```python
from build123d import *

# Parameters (mm, degrees)
SKETCH_3_R               = 2.5
SKETCH_3_R_2             = 1.375
SKETCH_3_R_3             = 0.625
EXTRUDE_1_DEPTH          = 12
CUT_EXTRUDE_START        = -6
SKETCH_4_R               = 1.375
SKETCH_4_R_2             = 0.625
CUT_EXTRUDE_1_DEPTH      = 6
CUT_EXTRUDE_2_DEPTH      = 6
CUT_EXTRUDE_3_DEPTH      = 98.323451249
CUT_EXTRUDE_3_DEPTH_BACK = 98.323451249
SKETCH_9_W               = 7.034569735
SKETCH_9_H               = 2.5


with BuildPart() as part:
    # 草图3 → 凸台-拉伸1 (new body)
    # profile 1 of 4: a face of its own
    with BuildSketch(Plane.XY):
        with BuildLine():
            ThreePointArc((-61.260434814, -42.25), (-62.911250508, -39.426764685), (-66.181254237, -39.480854503))
            Line((-66.181254237, -39.480854503), (-67.215081256, -40.482765899))
            ThreePointArc((-67.215081256, -40.482765899), (-66.804847725, -44.526501605), (-62.766497887, -44.986741313))
            ThreePointArc((-62.766497887, -44.986741313), (-61.661816101, -43.8118882), (-61.260434814, -42.25))
        make_face()
        with Locations((-64.5, -42.25)):
            Circle(SKETCH_3_R, mode=Mode.SUBTRACT)
    # profile 2 of 4: a face of its own
    with BuildSketch(Plane.XY):
        with BuildLine():
            ThreePointArc((-62.766497887, -44.986741313), (-66.804847725, -44.526501605), (-67.215081256, -40.482765899))
            Line((-67.215081256, -40.482765899), (-71.404577544, -44.542926834))
            Line((-71.404577544, -44.542926834), (-68.869512223, -46.563873564))
            ThreePointArc((-68.869512223, -46.563873564), (-68.283195443, -46.88782244), (-67.622796748, -47))
            Line((-67.622796748, -47), (-65.944900832, -47))
            Line((-65.944900832, -47), (-62.766497887, -44.986741313))
        make_face()
    # profile 3 of 4: a face of its own
    with BuildSketch(Plane.XY):
        with Locations((-78.5, -53.325)):
            Circle(SKETCH_3_R_2)
        with Locations((-78.5, -53.325)):
            Circle(SKETCH_3_R_3, mode=Mode.SUBTRACT)
    # profile 4 of 4: a face of its own
    with BuildSketch(Plane.XY):
        with BuildLine():
            Line((-68.869512223, -46.563873564), (-71.404577544, -44.542926834))
            Line((-71.404577544, -44.542926834), (-79.356399518, -52.24926543))
            ThreePointArc((-79.356399518, -52.24926543), (-77.902892111, -52.086417274), (-77.125, -53.325))
            ThreePointArc((-77.125, -53.325), (-77.295362144, -53.987927323), (-77.764232924, -54.486581598))
            Line((-77.764232924, -54.486581598), (-65.944900832, -47))
            Line((-65.944900832, -47), (-67.622796748, -47))
            ThreePointArc((-67.622796748, -47), (-68.283195443, -46.88782244), (-68.869512223, -46.563873564))
        make_face()
    extrude(amount=EXTRUDE_1_DEPTH)

    # 草图4 → 切除-拉伸1 (cut)
    with BuildSketch(Plane.XY.offset(6).offset(CUT_EXTRUDE_START)):
        with Locations((-78.5, -53.325)):
            Circle(SKETCH_4_R)
        with Locations((-78.5, -53.325)):
            Circle(SKETCH_4_R_2, mode=Mode.SUBTRACT)
    extrude(amount=CUT_EXTRUDE_1_DEPTH, mode=Mode.SUBTRACT)

    # 草图5 → 切除-拉伸2 (cut)
    with BuildSketch(Plane(origin=(0, 0, 0), x_dir=(-1, 0, 0), z_dir=(0, 0, -1))):
        with BuildLine():
            Line((79.356399518, -52.24926543), (78.605866383, -51.521902256))
            ThreePointArc((78.605866383, -51.521902256), (78.66209541, -51.603950043), (78.681882496, -51.701428318))
            ThreePointArc((78.681882496, -51.701428318), (78.612326251, -51.874460255), (78.442362088, -51.951208578))
            ThreePointArc((78.442362088, -51.951208578), (78.926279835, -52.017746963), (79.356399518, -52.24926543))
        make_face()
        with BuildLine():
            Line((79.691485429, -51.10916302), (78.328547162, -51.10916302))
            Line((78.328547162, -51.10916302), (78.328547162, -51.253144251))
            Line((78.328547162, -51.253144251), (78.605866383, -51.521902256))
            Line((78.605866383, -51.521902256), (79.356399518, -52.24926543))
            ThreePointArc((79.356399518, -52.24926543), (78.926279835, -52.017746963), (78.442362088, -51.951208578))
            ThreePointArc((78.442362088, -51.951208578), (78.385355708, -51.954787722), (78.328547162, -51.960731359))
            Line((78.328547162, -51.960731359), (78.328547162, -52.568011757))
            Line((78.328547162, -52.568011757), (79.691485429, -52.568011757))
            Line((79.691485429, -52.568011757), (79.691485429, -51.10916302))
        make_face()
        with BuildLine():
            Line((76.773632808, -53.859117327), (76.559713092, -53.723616657))
            Line((76.559713092, -53.723616657), (76.559713092, -54.626372146))
            Line((76.559713092, -54.626372146), (77.832544784, -54.626372146))
            Line((77.832544784, -54.626372146), (77.832544784, -53.006023906))
            Line((77.832544784, -53.006023906), (77.162510093, -53.006023906))
            ThreePointArc((77.162510093, -53.006023906), (77.125199423, -53.301582625), (77.152422696, -53.598240569))
            ThreePointArc((77.152422696, -53.598240569), (77.36758294, -54.104908073), (77.764232924, -54.486581598))
            Line((77.764232924, -54.486581598), (76.773632808, -53.859117327))
        make_face()
        with BuildLine():
            ThreePointArc((77.152422696, -53.598240569), (77.049210108, -53.853814684), (76.773632808, -53.859117327))
            Line((76.773632808, -53.859117327), (77.764232924, -54.486581598))
            ThreePointArc((77.764232924, -54.486581598), (77.36758294, -54.104908073), (77.152422696, -53.598240569))
        make_face()
    extrude(amount=-CUT_EXTRUDE_2_DEPTH, mode=Mode.SUBTRACT)

    # 草图9 → 切除-拉伸3 (cut, two sides: drawn at the far end of the back side and taken through both)
    with BuildSketch(Plane(origin=(-4.269265018, 5.396813566, 0), x_dir=(-0.784272958804573, -0.6204159299114752, 0), z_dir=(0.6204159299114752, -0.784272958804573, 0)).offset(-CUT_EXTRUDE_3_DEPTH_BACK)):
        with Locations((76.928026692, -1.25)):
            Rectangle(SKETCH_9_W, SKETCH_9_H)
        Polygon((74.298785761, -9.5), (73.410741824, -9.5), (73.410741824, -12), (80.445311559, -12), (80.445311559, -9.5), align=None)
    extrude(amount=CUT_EXTRUDE_3_DEPTH + CUT_EXTRUDE_3_DEPTH_BACK, mode=Mode.SUBTRACT)


solid = part.part
```
Verification items for the finished model (mm, model axes). A direction names the side the tool comes from. Coordinates: 2 decimals unless noted, no trailing zeros. Write each loop counter-clockwise with the first axis right and the second up, starting at its lowest first coordinate (ties: lowest second). Pieces come first, ordered by that corner, then holes. Notation, with made-up numbers: M 27,74.25 L 53,74.25 A25 cw 53,91.25 Z; hole C -23,12 d10. An arc over 180 degrees is marked long. One line per item, written item: value.
Item 1: Section check A-A, the plane x = -63.25. Record the boundary of the cut face in (y, z), plus the area to 3 significant figures.
Check sheet entries:
outline: M -45.29,2.5 L -44.42,2.5 L -44.42,9.5 L -45.29,9.5 Z; M -40.08,2.5 L -39.26,2.5 L -39.26,9.5 L -40.08,9.5 Z
area: 11.9 mm^2
Item 2: Access from +Z, -Z, +X, -X, +Y, -Y to the whole of each face (thin tool, end or side, straight path). Record for faces 1 (the flat face through (-67, -44, 9.5)), 2 (the flat face through (-66, -45, 2.5)), 3 (the flat face through (-72, -48, 0)).
Check sheet entries:
face 1: +Z, +X, +Y
face 2: -Z, +X, +Y
face 3: -Z, +X, -X, +Y, -Y
Item 3: Scan lines: line 1 along Y through (x, z) = (-64.5, 5); line 2 along Y through (x, z) = (-78.5, 8.3); line 3 along X through (y, z) = (-42.5, 4.25). Record each from-to range of solid material in increasing order.
Check sheet entries:
line 1: y = -46.08 to -44.75, -39.75 to -39.01
line 2: y = -54.7 to -53.95, -52.7 to -51.42
line 3: x = -69.3 to -66.99, -62.01 to -61.27
Item 4: Mould release check, pull along Y, two halves, no side actions. Record for faces 4 (the flat face through (-67.36, -44.51, 1.27)), 5 (the cylindrical face through (-79.637, -54.098, 8.958)), 6 (the cylindrical face through (-77.92, -53.56, 8.96)), 7 (the flat face through (-73, -48, 12)): pulls with the +Y half, pulls with the -Y half, needs draft (parallel to the pull), parting line crosses it, or undercut.
Check sheet entries:
face 4: pulls with the +Y half
face 5: parting line crosses it
face 6: undercut
face 7: needs draft
Item 5: Gauge pin test, flat ends, axial feed: pin 1 Ø2.5 at (x, y) = (-64, -44.5) entering from -Z; pin 2 Ø6 at (x, z) = (-74.5, 9.5) entering from -Y; pin 3 Ø5 at (x, z) = (-67.5, 3) entering from -Y. Record the tip position at first contact, or that the pin passes through.
Check sheet entries:
pin 1: stops at z = 2.5
pin 2: stops at y = -54.32
pin 3: stops at y = -49.57
Item 6: Section check B-B, the plane z = 7. State how many separate pieces and enclosed holes the cut face has, plus the area to 3 significant figures.
Check sheet entries:
separate pieces: 1
enclosed holes: 2
area: 80.6 mm^2
Item 7: Section check D-D, the plane y = -45.5. Record the boundary of the cut face in (x, z).
Check sheet entries:
outline: M -72.39,0 L -66.58,0 L -66.58,2.5 L -63.58,2.5 L -63.58,9.5 L -66.58,9.5 L -66.58,12 L -72.39,12 Z
